CAD build for the part. Positions are in the model's coordinates, mm. A direction names the side the tool comes from. Give positions to 0.01 mm unless a question says otherwise; leave off trailing zeros. Loops run counter-clockwise (first coordinate to the right, second up) from the corner with the lowest first, then second, coordinate; pieces in that order, holes last.
Item 1: Which spindle directions (+Z, -Z, +X, -X, +Y, -Y) get a long thin tool onto all of the face, cutting with end or side? Do faces 1 (the flat face through (14, 3.175, 243)), 2 (the flat face through (7, 2, 0)). Say none if no direction does.
Item 2: Drop flat-ended pins along their axis: P1, Ø6.5, axis at y = 15, z = 145.5, coming from the +X side (3 decimals); P2, Ø3, axis at x = 21.5, y = 6, coming from the -Z side; P3, Ø6.5, axis at x = 15.5, z = 267.5, coming from the +Y side (3 decimals). Give the stop position or say it passes through.
Item 3: Probe probe 1 along Z at (x, y) = (12.7, 1.15) (3 decimals); probe 2 along Z at (x, y) = (1.65, 12.7) (3 decimals); probe 3 along Y at (x, z) = (1.35, 12.7). List the from-to ranges inside material, lowest first.
Item 4: Saw through at B-B on x = 20. Give the cut face in (y, z) (3 decimals), plus the area to 3 significant figures.
Item 5: Saw through at A-A on z = 59.5. Give the cut face in (x, y) (3 decimals), plus the area to 3 significant figures.
Autodesk Inventor part; units mm, degrees
ref_plane "YZ Plane" through (0, 0, 0) normal (1, 0, 0) x (0, 1, 0)
ref_plane "XZ Plane" through (0, 0, 0) normal (0, 1, 0) x (-1, 0, 0)
ref_plane "XY Plane" through (0, 0, 0) normal (0, 0, 1) x (1, 0, 0)
sketch "Sketch1" plane through (0, 0, 0) normal (0, 0, 1) x (1, 0, 0)
  line L0 (0, 25.4) -> (0, 0)
  line L1 (0, 0) -> (25.4, 0)
  line L2 (3.175, 25.4) -> (3.175, 4.953)
  line L3 (4.953, 3.175) -> (25.4, 3.175)
  line L4 (0, 25.4) -> (3.175, 25.4)
  line L5 (25.4, 3.175) -> (25.4, 0)
  line L6 (3.175, 4.953) -> (3.175, 3.175)
  line L7 (4.953, 3.175) -> (3.175, 3.175)
  dimension "d0" = 25.4
  dimension "d1" = 25.4
  dimension "d2" = 3.175
extrude "Extrusion1" add sketch "Sketch1" along normal blind 492.125
sketch "Sketch7" plane through (3.175, 3.175, 0) normal (1, 0, 0) x (0, 0, -1)
  circle A0 centre (-479.425, 9.525) radius 2.8124
  line L0 (0, 22.225) -> (-492.125, 22.225)
  line L1 (-492.125, 0) -> (-492.125, 22.225)
  circle A1 centre (-12.7, 9.525) radius 2.8124
  point P0 (0, -3.175)
  dimension "d43" = 12.7
  dimension "d44" = 12.7
  dimension "d47" = 466.725
hole "Hole4" at (3.175, 12.7, 479.425) at (3.175, 12.7, 12.7) direction (-1, 0, 0) diameter 6.7564 depth 25.4 tip angle 118
sketch "Sketch8" plane through (3.175, 3.175, 0) normal (0, 1, 0) x (1, 0, 0)
  circle A0 centre (9.525, -339.725) radius 5.1637
  line L0 (22.225, 0) -> (22.225, -492.125)
  line L1 (22.225, -492.125) -> (0, -492.125)
  point P0 (-3.175, 0)
  dimension "d59" = 12.7
  dimension "d60" = 152.4
hole "Hole5" at (12.7, 3.175, 339.725) direction (0, -1, 0) diameter 6.7564 depth 25.4 tip angle 118
sketch "Sketch9" plane through (3.175, 3.175, 0) normal (0, 1, 0) x (1, 0, 0)
  circle A0 centre (9.525, -152.4) radius 4.6363
  line L0 (22.225, 0) -> (22.225, -492.125)
  line L1 (22.225, 0) -> (0, 0)
  point P0 (-3.175, 0)
  dimension "d68" = 12.7
  dimension "d69" = 152.4
hole "Hole6" at (12.7, 3.175, 152.4) direction (0, -1, 0) diameter 6.7564 depth 25.4 tip angle 118
Results below:
1. face 1: +Z, -Z, +X, +Y
1. face 2: -Z, +X, -X, +Y, -Y
2. P1: stops at x = 3.175
2. P2: passes through
2. P3: stops at y = 3.175
3. probe 1: z = 0 to 149.022, 155.778 to 336.347, 343.103 to 492.125
3. probe 2: z = 0 to 9.322, 16.078 to 476.047, 482.803 to 492.125
3. probe 3: y = 0 to 9.32, 16.08 to 25.4
4. outline: (0, 0) - (3.175, 0) - (3.175, 492.125) - (0, 492.125) - close
4. area: 1,560 mm2
5. outline: (0, 0) - (25.4, 0) - (25.4, 3.175) - (3.175, 3.175) - (3.175, 25.4) - (0, 25.4) - close
5. area: 151 mm2
